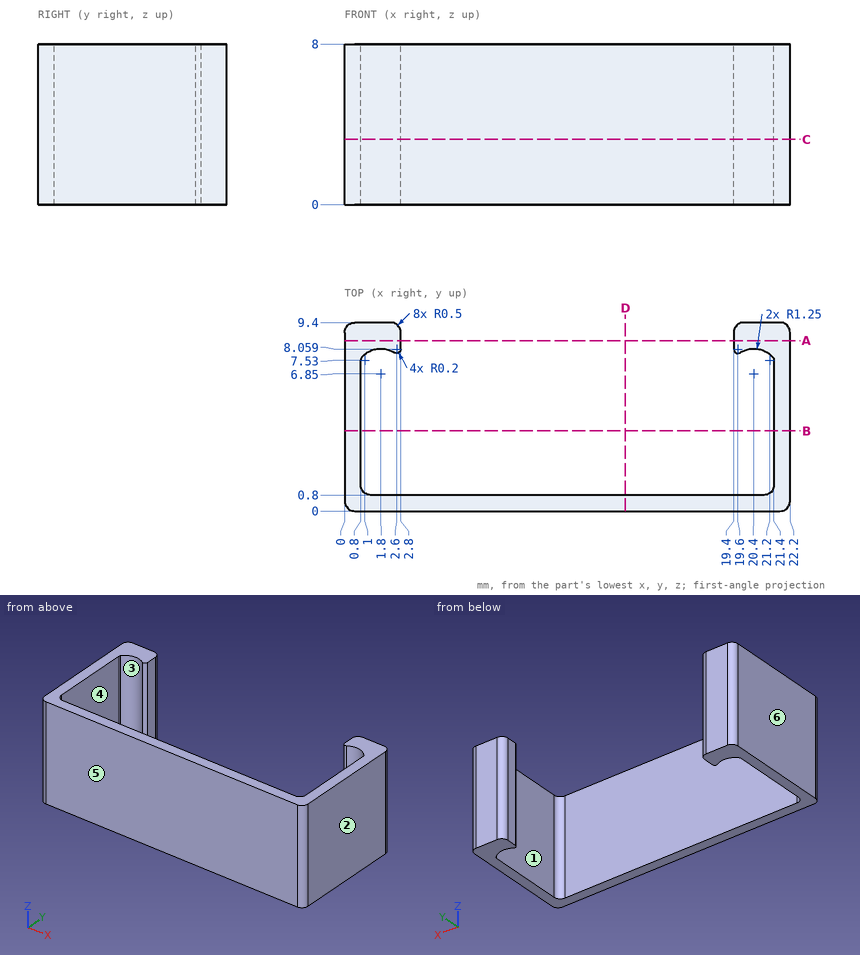
Here's the drawing with two shaded views (mm, measured from the low corner). I have some questions. A direction names the side the tool comes from. Coordinates: 2 decimals unless noted, no trailing zeros. Loops run counter-clockwise (first coordinate to the right, second up) from the corner with the lowest first, then second, coordinate; pieces in that order, holes last. Notation, with made-up numbers: (68.5, -29.75) - (100.5, -29.75) arc R21 cw to (100.5, -7.75) - close; hole circle Ø3 at (61.25, -24). An arc over 180 degrees is marked (long way). Answer as CSV lines item,"result". Start each with the question number.
1) Which directions (+Z, -Z, +X, -X, +Y, -Y) give clear straight access to the entire face, cutting with the end or side of a thin tool? Please do the marked faces 1 and 2.
2) I need wall thicknesses on line 1 (X direction, y = 7.25, z = 1.25); line 2 (Y direction, x = 1.5, z = 3.75); line 3 (X direction, y = 8.75, z = 3.25). Which ranges of each line are inside material? Lowest first, please. Write a range as from..to.
3) Suppose I cut it at B-B (y = 4). Please give me the cut outline in (x, z).
4) Suppose I cut it at C-C (z = 3.25). Please give me the cut outline in (x, y).
5) Suppose I cut it at D-D (x = 14). Please give me the cut outline in (y, z).
6) Suppose I cut it at A-A (y = 8.5). Please give me the cut outline in (x, z), plus the area to 3 significant figures.
7) Thinking about a two-plate mould opening in X: for the marked faces 3, 4, 5 and 6, which applies, pulls with the +X half, pulls with the -X half, needs draft (parallel to the pull), parting line crosses it, or undercut?
Check result:
1,face 1,"+Z, -Z"
1,face 2,"+Z, -Z, +X, +Y, -Y"
2,line 1,"x = 0..0.8, 21.4..22.2"
2,line 2,"y = 0..0.8, 8.06..9.4"
2,line 3,"x = 0..2.8, 19.4..22.2"
3,outline,"(0, 0) - (0.8, 0) - (0.8, 8) - (0, 8) - close; (21.4, 0) - (22.2, 0) - (22.2, 8) - (21.4, 8) - close"
4,outline,"(0, 0.5) arc R0.5 ccw to (0.5, 0) - (21.7, 0) arc R0.5 ccw to (22.2, 0.5) - (22.2, 8.9) arc R0.5 ccw to (21.7, 9.4) - (19.9, 9.4) arc R0.5 ccw to (19.4, 8.9) - (19.4, 8.06) arc R0.2 ccw to (19.71, 7.89) arc R1.25 cw to (21.35, 7.66) arc R0.2 cw to (21.4, 7.53) - (21.4, 1.3) arc R0.5 cw to (20.9, 0.8) - (1.3, 0.8) arc R0.5 cw to (0.8, 1.3) - (0.8, 7.53) arc R0.2 cw to (0.85, 7.66) arc R1.25 cw to (2.49, 7.89) arc R0.2 ccw to (2.8, 8.06) - (2.8, 8.9) arc R0.5 ccw to (2.3, 9.4) - (0.5, 9.4) arc R0.5 ccw to (0, 8.9) - close"
5,outline,"(0, 0) - (0.8, 0) - (0.8, 8) - (0, 8) - close"
6,outline,"(0, 0) - (2.8, 0) - (2.8, 8) - (0, 8) - close; (19.4, 0) - (22.2, 0) - (22.2, 8) - (19.4, 8) - close"
6,area,"44.8 mm²"
7,face 3,"undercut"
7,face 4,"undercut"
7,face 5,"needs draft"
7,face 6,"pulls with the -X half"
